Geometry: final body of the model. Coordinates: model frame, mm. A direction names the side the tool comes from. Give positions to 0.01 mm unless a question says otherwise; leave off trailing zeros. Write each loop counter-clockwise with the first axis right and the second up, starting at its lowest first coordinate (ties: lowest second). Pieces come first, ordered by that corner, then holes. Notation, with made-up numbers: (-24, 79) -> (17, 79) arc R17 cw to (17, 84) -> close; hole circle Ø6 at (72.25, 81). An arc over 180 degrees is marked (long way). Use CSV: the item, a comma, the result in double quotes. Start each with the question number.
1) Material intervals for line 1 (Y direction, x = 10, z = 46.5); line 2 (X direction, y = -5, z = 21.5) (3 decimals); line 3 (Y direction, x = 2.75, z = -11), sorted ascending. Write a range as [from, to].
2) Section D-D (z = -41). Count the separate pieces of the cut face and the enclosed holes in it, plus the area to 3 significant figures.
3) Section A-A (y = -6). Output: boundary loops of the cut face in (x, z) (3 decimals).
4) Section C-C (y = 21). Output: boundary loops of the cut face in (x, z) (3 decimals), plus the area to 3 significant figures.
5) Contact query for a flat-ended pin moving along its axis: P1, Ø3, axis at y = -12.7, z = -9.525, coming from the -X side. Output: stop coordinate, or through.
6) Section B-B (x = -3.75). Output: boundary loops of the cut face in (y, z) (3 decimals), plus the area to 3 significant figures.
7) Draft query along Z for faces 1 (the face through (11.684, 22, 1)), 2 (the face through (-11.13, -11.94, -37.35)). Return one class per face: pulls with the +Z half, pulls with the -Z half, needs draft (parallel to the pull), parting line crosses it, or undercut.
8) Set-up query: faces 3 (the face through (11.09, 13.46, -37.35)), 4 (the face through (-11.684, 22, 1)). Return all of +Z, -Z, +X, -X, +Y, -Y with unobstructed straight access to the full face (end or side cutting, diameter ignored); none if empty.
```python
from build123d import *

# Parameters (mm, degrees)
SKETCH1_W                                = 50.8
SKETCH1_H                                = 107.95
BOSS_EXTRUDE1_DEPTH                      = 25.4
CUT_EXTRUDE9_DEPTH                       = 108.95
MIRROR1_AT_THE_SECOND_PLANE_COPY_1_DEPTH = 108.95
CUT_EXTRUDE11_START                      = -26.4
SKETCH17_R                               = 2.54
CUT_EXTRUDE11_DEPTH                      = 27.4
SKETCH18_R                               = 2.54
CUT_EXTRUDE12_DEPTH                      = 51.8
LPATTERN1_COUNT                          = 9
LPATTERN1_PITCH                          = 12.7
LPATTERN2_COUNT                          = 9
LPATTERN2_PITCH                          = 12.7
LPATTERN2_COUNT_DIR2                     = 3
LPATTERN2_PITCH_DIR2                     = 12.7
FILLET1_R                                = 0.127


with BuildPart() as part:
    # Sketch1 → Boss-Extrude1 (new body)
    with BuildSketch(Plane(origin=(-12.7, 0, 0), x_dir=(0, -1, 0), z_dir=(-1, 0, 0))):
        Rectangle(SKETCH1_W, SKETCH1_H)
    extrude(amount=-BOSS_EXTRUDE1_DEPTH)

    # Sketch10 → Cut-Extrude9 (cut, through all)
    with BuildSketch(Plane.XY.offset(53.975)):
        with BuildLine():
            Line((-11.684, 24.384), (-11.684, 19.297089026))
            ThreePointArc((-11.684, 19.297089026), (-11.177055919, 18.630604499), (-10.39941737, 18.941204261))
            ThreePointArc((-10.39941737, 18.941204261), (-8.576144596, 21.276144596), (-6.241204261, 23.09941737))
            ThreePointArc((-6.241204261, 23.09941737), (-5.930604499, 23.877055919), (-6.597089026, 24.384))
            Line((-6.597089026, 24.384), (-11.684, 24.384))
        make_face()
        with BuildLine():
            Line((0, 24.384), (-4.8895, 24.384))
            Line((-4.8895, 24.384), (-4.8895, 22.679000251))
            ThreePointArc((-4.8895, 22.679000251), (-7.514726072, 20.886363558), (-9.525, 18.42381265))
            Line((-9.525, 18.42381265), (-9.525, 0))
            Line((-9.525, 0), (0, 0))
            Line((0, 0), (0, 24.384))
        make_face()
    cut_extrude9 = extrude(amount=-CUT_EXTRUDE9_DEPTH, mode=Mode.SUBTRACT)

    # Mirror1: Cut-Extrude9 across plane
    add(cut_extrude9.mirror(Plane.ZX), mode=Mode.SUBTRACT)

    # Mirror1 at the second plane: Cut-Extrude9 across plane
    add(cut_extrude9.mirror(Plane(origin=(0, 0, 0), x_dir=(0, 0, 1), z_dir=(1, 0, 0))), mode=Mode.SUBTRACT)

    # Mirror1 at the second plane copy 1 sketc → Mirror1 at the second plane copy 1 (cut, through all)
    with BuildSketch(Plane(origin=(0, 0, 53.975), x_dir=(-1, 0, 0), z_dir=(0, 0, 1))):
        with BuildLine():
            Line((-11.684, 24.384), (-11.684, 19.297089026))
            ThreePointArc((-11.684, 19.297089026), (-11.177055919, 18.630604499), (-10.39941737, 18.941204261))
            ThreePointArc((-10.39941737, 18.941204261), (-8.576144596, 21.276144596), (-6.241204261, 23.09941737))
            ThreePointArc((-6.241204261, 23.09941737), (-5.930604499, 23.877055919), (-6.597089026, 24.384))
            Line((-6.597089026, 24.384), (-11.684, 24.384))
        make_face()
        with BuildLine():
            Line((0, 24.384), (-4.8895, 24.384))
            Line((-4.8895, 24.384), (-4.8895, 22.679000251))
            ThreePointArc((-4.8895, 22.679000251), (-7.514726072, 20.886363558), (-9.525, 18.42381265))
            Line((-9.525, 18.42381265), (-9.525, 0))
            Line((-9.525, 0), (0, 0))
            Line((0, 0), (0, 24.384))
        make_face()
    extrude(amount=-MIRROR1_AT_THE_SECOND_PLANE_COPY_1_DEPTH, mode=Mode.SUBTRACT)

    # Sketch17 → Cut-Extrude11 (cut)
    with BuildSketch(Plane(origin=(12.7, 0, 0), x_dir=(0, 0, -1), z_dir=(1, 0, 0)).offset(CUT_EXTRUDE11_START)):
        with Locations((-41.275, 12.7)):
            Circle(SKETCH17_R)
    cut_extrude11 = extrude(amount=CUT_EXTRUDE11_DEPTH, mode=Mode.SUBTRACT)

    # Sketch18 → Cut-Extrude12 (cut, through all)
    with BuildSketch(Plane(origin=(0, 25.4, 0), x_dir=(1, 0, 0), z_dir=(0, 1, 0))):
        with Locations((0, -41.275)):
            Circle(SKETCH18_R)
    cut_extrude12 = extrude(amount=-CUT_EXTRUDE12_DEPTH, mode=Mode.SUBTRACT)

    # LPattern1: Cut-Extrude12 ×9
    with Locations(*[(0, 0, -i * LPATTERN1_PITCH) for i in range(1, LPATTERN1_COUNT)]):
        add(cut_extrude12, mode=Mode.SUBTRACT)

    # LPattern2: Cut-Extrude11 9 × 3
    with Locations(*[(0, -j * LPATTERN2_PITCH_DIR2, -i * LPATTERN2_PITCH) for i in range(LPATTERN2_COUNT) for j in range(LPATTERN2_COUNT_DIR2) if (i, j) != (0, 0)]):
        add(cut_extrude11, mode=Mode.SUBTRACT)

    # Fillet1
    fillet1_edges = [part.edges().sort_by_distance(p)[0] for p in [
        (-4.8895, -24.384, 0),
        (-4.8895, -22.679000251, 0),
        (-9.525, -18.42381265, 0),
        (4.8895, -22.679000251, 0),
        (4.8895, -24.384, 0),
        (9.525, -18.42381265, 0),
        (-4.8895, 22.679000251, 0),
        (-4.8895, 24.384, 0),
        (-9.525, 18.42381265, 0),
        (4.8895, 24.384, 0),
        (4.8895, 22.679000251, 0),
        (9.525, 18.42381265, 0),
    ]]
    fillet(fillet1_edges, radius=FILLET1_R)


solid = part.part
```
Answers follow:
1,line 1,"y = [-25.4, -24.38], [-19.56, 19.56], [24.38, 25.4]"
1,line 2,"x = [-12.7, -9.525], [9.525, 12.7]"
1,line 3,"y = [-25.4, -24.38], [24.38, 25.4]"
2,separate pieces,"1"
2,enclosed holes,"5"
2,area,"344 mm^2"
3,outline,"(-12.7, -53.975) -> (-9.525, -53.975) -> (-9.525, 53.975) -> (-12.7, 53.975) -> close; (9.525, -53.975) -> (12.7, -53.975) -> (12.7, 53.975) -> (9.525, 53.975) -> close"
4,outline,"(-12.7, -53.975) -> (-11.684, -53.975) -> (-11.684, 53.975) -> (-12.7, 53.975) -> close; (-8.844, -53.975) -> (-7.389, -53.975) -> (-7.389, 53.975) -> (-8.844, 53.975) -> close; (7.389, -53.975) -> (8.844, -53.975) -> (8.844, 53.975) -> (7.389, 53.975) -> close; (11.684, -53.975) -> (12.7, -53.975) -> (12.7, 53.975) -> (11.684, 53.975) -> close"
4,area,"533 mm^2"
5,P1,"passes through"
6,outline,"(-25.4, -53.975) -> (-24.384, -53.975) -> (-24.384, 53.975) -> (-25.4, 53.975) -> close; (24.384, -53.975) -> (25.4, -53.975) -> (25.4, 53.975) -> (24.384, 53.975) -> close"
6,area,"219 mm^2"
7,face 1,"needs draft"
7,face 2,"undercut"
8,face 3,"+X, -X"
8,face 4,"+Z, -Z"
